For this review, take the finished solid that the model builds, in its own axes (mm). Face numbers are marked on the shaded views. A direction names the side the tool comes from. Round coordinates to 2 decimals unless told otherwise and drop trailing zeros. Order: outer loops, then holes, each group sorted by start corner. A loop starts at its lowest first (then second) coordinate and runs counter-clockwise, first axis right, second up. Notation, with made-up numbers: M 70,-9 L 95,-9 A24 cw 95,20 Z; hole C -16,78 d2. An arc over 180 degrees is marked long. Use a Markdown table: item, result.
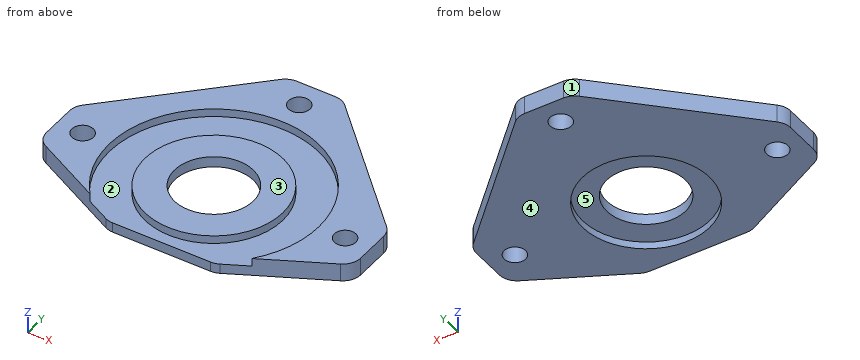
from build123d import *

# Parameters (mm, degrees)
F0_R     = 6
F1_DEPTH = 10
F2_R     = 35.5
F3_DEPTH = 4
F4_R     = 58.5
F4_R_2   = 38.5
F5_DEPTH = 4.5
F6_R     = 22
F7_DEPTH = 10.001


with BuildPart() as f1:
    # F0 (on Top) → F1 (new body)
    with BuildSketch(Plane.XY):
        with BuildLine():
            ThreePointArc((-85.071068, 17.928932), (-87.238795, 14.684699), (-88, 10.857864))
            Line((-88, 10.857864), (-88, -8.905047))
            ThreePointArc((-88, -8.905047), (-86.538952, -14.109498), (-82.582739, -17.793158))
            Line((-82.582739, -17.793158), (-31.972211, -43.88811))
            ThreePointArc((-31.972211, -43.88811), (-29.747321, -44.718053), (-27.389472, -45))
            Line((-27.389472, -45), (0, -45))
            Line((0, -45), (27.389472, -45))
            ThreePointArc((27.389472, -45), (29.747321, -44.718053), (31.972211, -43.88811))
            Line((31.972211, -43.88811), (82.582739, -17.793158))
            ThreePointArc((82.582739, -17.793158), (86.538952, -14.109498), (88, -8.905047))
            Line((88, -8.905047), (88, 10.857864))
            ThreePointArc((88, 10.857864), (87.238795, 14.684699), (85.071068, 17.928932))
            Line((85.071068, 17.928932), (17.928932, 85.071068))
            ThreePointArc((17.928932, 85.071068), (14.684699, 87.238795), (10.857864, 88))
            Line((10.857864, 88), (-10.857864, 88))
            ThreePointArc((-10.857864, 88), (-14.684699, 87.238795), (-17.928932, 85.071068))
            Line((-17.928932, 85.071068), (-85.071068, 17.928932))
        make_face()
        with Locations((-73.5, 0)):
            Circle(F0_R, mode=Mode.SUBTRACT)
        with Locations((73.5, 0)):
            Circle(F0_R, mode=Mode.SUBTRACT)
        with Locations((0, 73.5)):
            Circle(F0_R, mode=Mode.SUBTRACT)
    extrude(amount=F1_DEPTH)

    # F2 (on face) → F3 (cut)
    with BuildSketch(Plane(origin=(0, 0, 0), x_dir=(1, 0, 0), z_dir=(0, 0, -1))):
        Circle(F2_R)
    extrude(amount=-F3_DEPTH, mode=Mode.SUBTRACT)

    # F4 (on face) → F5 (cut)
    with BuildSketch(Plane.XY.offset(10)):
        Circle(F4_R)
        Circle(F4_R_2, mode=Mode.SUBTRACT)
    extrude(amount=-F5_DEPTH, mode=Mode.SUBTRACT)

    # F6 (on face) → F7 (cut, through all)
    with BuildSketch(Plane.XY.offset(10)):
        Circle(F6_R)
    extrude(amount=-F7_DEPTH, mode=Mode.SUBTRACT)


solid = f1.part
Q1. Add section A-A (y = 73.5). Write out the cut boundary in (x, z).
Determined:
| item | result |
|---|---|
| outline | M -29.5,0 L -6,0 L -6,10 L -29.5,10 Z; M 6,0 L 29.5,0 L 29.5,10 L 6,10 Z |
Q2. Clearance check with flat-ended pins moving along their axes: pin 1 (19 mm diameter, centred on x = -73.5, y = 0, fed in from +Z); pin 2 (5 mm diameter, centred on x = -65, z = 3, fed in from -Y); pin 3 (3 mm diameter, centred on y = 30, z = 6, fed in from +X); pin 4 (5 mm diameter, centred on y = 23, z = 7.5, fed in from -X). State where each tip first meets the part, or that it passes through.
Determined:
| item | result |
|---|---|
| pin 1 | stops at z = 10 |
| pin 2 | stops at y = -28.15 |
| pin 3 | stops at x = 74.5 |
| pin 4 | stops at x = -82.5 |
Q3. Add section B-B (y = 0). Write out the cut boundary in (x, z), then the cut area to 3 significant figures.
Determined:
| item | result |
|---|---|
| outline | M -88,0 L -79.5,0 L -79.5,10 L -88,10 Z; M -67.5,0 L -35.5,0 L -35.5,4 L -22,4 L -22,10 L -38.5,10 L -38.5,5.5 L -58.5,5.5 L -58.5,10 L -67.5,10 Z; M 22,4 L 35.5,4 L 35.5,0 L 67.5,0 L 67.5,10 L 58.5,10 L 58.5,5.5 L 38.5,5.5 L 38.5,10 L 22,10 Z; M 79.5,0 L 88,0 L 88,10 L 79.5,10 Z |
| area | 792 mm^2 |
Q4. Wall thickness on line 1 along X through (y, z) = (0.5, 2.5); line 2 along X through (y, z) = (-0.5, 6); line 3 along X through (y, z) = (17.5, 8): over which ranges is each line inside the solid? List them lowest first. Write a range as [from, to].
Determined:
| item | result |
|---|---|
| line 1 | x = [-88, -79.48], [-67.52, -35.5], [35.5, 67.52], [79.48, 88] |
| line 2 | x = [-88, -79.48], [-67.52, -58.5], [-38.5, -21.99], [21.99, 38.5], [58.5, 67.52], [79.48, 88] |
| line 3 | x = [-85.48, -55.82], [-34.29, -13.33], [13.33, 34.29], [55.82, 85.48] |
Q5. Add section C-C (z = 2.5). Write out the cut boundary in (x, y).
Determined:
| item | result |
|---|---|
| outline | M -88,-8.91 A10 ccw -82.58,-17.79 L -31.97,-43.89 A10 ccw -27.39,-45 L 27.39,-45 A10 ccw 31.97,-43.89 L 82.58,-17.79 A10 ccw 88,-8.91 L 88,10.86 A10 ccw 85.07,17.93 L 17.93,85.07 A10 ccw 10.86,88 L -10.86,88 A10 ccw -17.93,85.07 L -85.07,17.93 A10 ccw -88,10.86 Z; hole C -73.5,0 d12; hole C 0,0 d71; hole C 0,73.5 d12; hole C 73.5,0 d12 |
Q6. Draft analysis for pull direction X (two halves, no side actions). For the marked faces 1, 2 and 3, state which applies: pulls with the +X half, pulls with the -X half, needs draft (parallel to the pull), parting line crosses it, or undercut.
Determined:
| item | result |
|---|---|
| face 1 | pulls with the -X half |
| face 2 | undercut |
| face 3 | needs draft |
Q7. Machinability: for the marked faces 4 and 5, which of the approach directions +Z, -Z, +X, -X, +Y, -Y give a long, thin tool a straight path to every point of the face, cutting with its end or side? Answer none if there is none.
Determined:
| item | result |
|---|---|
| face 4 | -Z, +X, -X, +Y, -Y |
| face 5 | -Z |
Q8. Add section D-D (x = -74). Write out the cut boundary in (y, z).
Determined:
| item | result |
|---|---|
| outline | M -22.22,0 L -5.98,0 L -5.98,10 L -22.22,10 Z; M 5.98,0 L 29,0 L 29,10 L 5.98,10 Z |
